The listing builds one solid part. Answer for the finished solid, in the listing's coordinates (mm). A direction names the side the tool comes from. Round coordinates to 2 decimals unless told otherwise and drop trailing zeros. Write each loop counter-clockwise with the first axis right and the second up, starting at its lowest first coordinate (ties: lowest second). Pieces come first, ordered by that corner, then holes. Notation, with made-up numbers: (-8.75, 69.5) - (6.25, 69.5) arc R17 ccw to (6.25, 73.5) - close; hole circle Ø5 at (36.5, 17.5). An arc over 180 degrees is marked (long way). Return JSON: item names as keys, results as strings. Group by question number.
from build123d import *

# Parameters (mm, degrees)
SKETCH_1_W          = 10.2
SKETCH_1_H          = 6
EXTRUDE_1_DEPTH     = 3.3
EXTRUDE_START       = 3.3
EXTRUDE_2_DEPTH     = 1.2
CUT_EXTRUDE_2_DEPTH = 13.660568708
SKETCH_2_5_R        = 2
CUT_EXTRUDE_4_DEPTH = 13.660568708


with BuildPart() as part:
    # 草图1 → 凸台-拉伸1 (new body)
    with BuildSketch(Plane(origin=(0, 0, 0), x_dir=(1, 0, 0), z_dir=(0, 1, 0))):
        with Locations((5.1, 3)):
            Rectangle(SKETCH_1_W, SKETCH_1_H)
    extrude(amount=EXTRUDE_1_DEPTH)

    # 草图2 → 凸台-拉伸2 (add)
    with BuildSketch(Plane(origin=(0, 0, 0), x_dir=(1, 0, 0), z_dir=(0, 1, 0)).offset(EXTRUDE_START)):
        with BuildLine():
            Line((2.1, 3), (2.1, 0))
            Line((2.1, 0), (5.1, 0))
            ThreePointArc((5.1, 0), (7.221320344, 0.878679656), (8.1, 3))
            Line((8.1, 3), (8.1, 6))
            Line((8.1, 6), (5.1, 6))
            ThreePointArc((5.1, 6), (2.978679656, 5.121320344), (2.1, 3))
        make_face()
    extrude(amount=EXTRUDE_2_DEPTH)

    # 草图3 → 切除-拉伸2 (cut, through all)
    with BuildSketch(Plane.XY):
        Polygon((0, 2.1), (2.1, 0), (0, 0), align=None)
        Polygon((8.1, 0), (10.2, 2.1), (10.2, 0), align=None)
    extrude(amount=-CUT_EXTRUDE_2_DEPTH, mode=Mode.SUBTRACT)

    # 草图2<5> → 切除-拉伸4 (cut, through all)
    with BuildSketch(Plane(origin=(0, 0, 0), x_dir=(1, 0, 0), z_dir=(0, 1, 0))):
        with Locations(Location((5.1, 3, 0), (0, 0, 270))):
            Circle(SKETCH_2_5_R)
    extrude(amount=CUT_EXTRUDE_4_DEPTH, mode=Mode.SUBTRACT)


solid = part.part
(1) Find section B-B (z = -3.5). Write down the section's boundary in (x, y).
(2) Flat-ended cylindrical pins translate along their axes: pin 1 (3 mm diameter, centred on x = 8.5, z = -1, fed in from +Y); pin 2 (1.3 mm diameter, centred on y = 4, z = -4, fed in from +X). Find the tip coordinate at first contact, or state that the pin passes through.
(3) For faces 1 (the cylindrical face through (3, 3.89, -5.14)), 2 (the cylindrical face through (7.2, 3.89, -0.86)), 3 (the flat face through (8.1, 4, -4)), determine the directions among +Z, -Z, +X, -X, +Y, -Y from which every point of the face is accessible in a straight line to the end or side of a thin tool.
(4) Determine the mould class of faces 4 (the cylindrical face through (3.148, 2.218, -3.434)), 5 (the flat face through (9, 3.3, -3)), 6 (the flat face through (1, 1.1, -3)), 7 (the flat face through (9.1, 1, -3)) for opening direction X: +X half, -X half, draft (parallel to the pull), parting line (faces both ways), or undercut.
(5) Find section D-D (y = 1.9). Write down the section's boundary in (x, z), plus the area to 3 significant figures.
(6) Find section A-A (y = 4.15). Write down the section's boundary in (x, z).
(7) Find section C-C (x = 6.5). Write down the section's boundary in (y, z).
(8) Consider line 1 (Z direction, x = 5.1, y = 1.7); line 2 (X direction, y = 3.1, z = -3); line 3 (Z direction, x = 4, y = 3.6). Determine where each line is inside the solid, lowest interval first.
Check sheet entries:
{
 "1": {"outline": "(0, 2.1) - (2.1, 0) - (3.16, 0) - (3.16, 4.5) - (2.14, 4.5) - (2.14, 3.3) - (0, 3.3) - close; (7.04, 0) - (8.1, 0) - (10.2, 2.1) - (10.2, 3.3) - (8.1, 3.3) - (8.1, 4.5) - (7.04, 4.5) - close"},
 "2": {"pin 1": "stops at y = 4.5", "pin 2": "stops at x = 8.1"},
 "3": {"face 1": "-Z, -X, +Y", "face 2": "+Z, +X, +Y", "face 3": "+Z, -Z, +X, +Y"},
 "4": {"face 4": "undercut", "face 5": "draft", "face 6": "-X half", "face 7": "+X half"},
 "5": {"outline": "(0.2, -6) - (10, -6) - (10, 0) - (0.2, 0) - close; hole circle Ø4 at (5.1, -3)", "area": "46.2 mm^2"},
 "6": {"outline": "(2.1, -3) arc R3 ccw to (5.1, -6) - (8.1, -6) - (8.1, -3) arc R3 ccw to (5.1, 0) - (2.1, 0) - close; hole circle Ø4 at (5.1, -3)"},
 "7": {"outline": "(0, -6) - (4.5, -6) - (4.5, -4.43) - (0, -4.43) - close; (0, -1.57) - (4.5, -1.57) - (4.5, -0.35) - (3.3, -0.35) - (3.3, 0) - (0, 0) - close"},
 "8": {"line 1": "z = -6 to -5, -1 to 0", "line 2": "x = 0 to 3.1, 7.1 to 10.2", "line 3": "z = -5.79 to -4.67, -1.33 to 0"}
}
